```python
from build123d import *

# Parameters (mm, degrees)
F0_R     = 15
F1_DEPTH = 10
F2_SIZE  = 1
F4_D     = 5


with BuildPart() as f1:
    # F0 (on Top) → F1 (new body)
    with BuildSketch(Plane.XY):
        Circle(F0_R)
    extrude(amount=F1_DEPTH)

    # F2
    f2_edges = [f1.edges().sort_by_distance(p)[0] for p in [
        (-15, 0, 10),
        (-15, 0, 0),
    ]]
    chamfer(f2_edges, length=F2_SIZE)

    # F4 (through all)
    with Locations(Plane.XY.offset(10)):
        with Locations((0, 0)):
            Hole(F4_D / 2)


solid = f1.part
```
Can you work these out from the model? Positions are in its coordinate system, mm. Give positions to 0.01 mm unless a question says otherwise; leave off trailing zeros. Write each loop counter-clockwise with the first axis right and the second up, starting at its lowest first coordinate (ties: lowest second). Pieces come first, ordered by that corner, then holes. Notation, with made-up numbers: (45.25, 8) - (66.25, 8) arc R28 cw to (66.25, 39) - close; hole circle Ø4 at (89.5, 24). An arc over 180 degrees is marked (long way). Write item = value, one per line. Start each with the question number.
1. Imagine slicing it at C-C (z = 8.25). Please give me the cut outline in (x, y).
2. Imagine slicing it at A-A (x = 0). Please give me the cut outline in (y, z), and give its area (3 significant figures).
3. Thinking about a two-plate mould opening in X: for faces 1 (the face through (0, -3, 0)), 2 (the face through (0.54, -2.44, 4.93)), 3 (the face through (-14.985, 0.66, 4.944)), which applies, released by +X, released by -X, zero draft, split by the parting line, or undercut?
4. Please list where these lines run through material, in increasing order: line 1 (Y direction, x = 0, z = 6.25); line 2 (X direction, y = 1, z = 4.25); line 3 (X direction, y = -2.25, z = 7.75).
5. For pin 1 (3 mm diameter, centred on x = 0, y = 0, fed in from +Z); pin 2 (2 mm diameter, centred on x = 2.5, z = 7.5, fed in from -Y); pin 3 (4 mm diameter, centred on x = 3, z = 7.5, fed in from +Y); pin 4 (3 mm diameter, centred on x = 4, z = 9, fed in from +Y), each with a flat end and sliding along its axis, tell me the tip position at first contact or that it passes through.
Worked answers:
q1.outline = circle Ø30 at (0, 0); hole circle Ø5 at (0, 0)
q2.outline = (-15, 1) - (-14, 0) - (-2.5, 0) - (-2.5, 10) - (-14, 10) - (-15, 9) - close; (2.5, 0) - (14, 0) - (15, 1) - (15, 9) - (14, 10) - (2.5, 10) - close
q2.area = 248 mm2
q3.face_1 = zero draft
q3.face_2 = undercut
q3.face_3 = split by the parting line
q4.line_1 = -15 to -2.5, 2.5 to 15
q4.line_2 = -14.97 to -2.29, 2.29 to 14.97
q4.line_3 = -14.83 to -1.09, 1.09 to 14.83
q5.pin_1 = through
q5.pin_2 = -14.92
q5.pin_3 = 14.97
q5.pin_4 = 14.79
